CAD build for the part. Positions are in the model's coordinates, mm. Coordinates: 2 decimals unless noted, no trailing zeros.
1) Wall check: line 1 along X through (y, z) = (8, 0.3); line 2 along Y through (x, z) = (11, 2.3); line 3 along X through (y, z) = (83, 2.3). Give the ranges that are in metal, low to high.
2) Pin check, flat tips, straight feed: pin 1 Ø6 at (x, y) = (99.695, 80.645) entering from +Z; pin 2 Ø3.5 at (x, y) = (99.695, 8.255) entering from +Z; pin 3 Ø5 at (x, y) = (8.255, 80.645) entering from +Z. Stop position of each tip, or through.
3) Two-plate mould, pull along Y, no slides. Class faces 1 (the cylindrical face through (1.449, 87.372, 1.61)), 2 (the cylindrical face through (8.7, 78.8, 0.4)), 3 (the cylindrical face through (1.449, 1.528, 1.61)), 4 (the cylindrical face through (101.094, 9.538, 0.431)): +Y half, -Y half, draft (parallel to the pull), parting line (faces both ways), or undercut.
```python
from build123d import *

# Parameters (mm, degrees)
F0_W           = 107.95
F0_H           = 88.9
F1_DEPTH       = 3.175
F3_D           = 3.7973
F3_CSINK_D     = 7.7978
F3_CSINK_ANGLE = 82
F4_R           = 5.08


with BuildPart() as f1:
    # F0 (on Top) → F1 (new body)
    with BuildSketch(Plane.XY):
        with Locations((53.975, 44.45)):
            Rectangle(F0_W, F0_H)
    extrude(amount=F1_DEPTH)

    # F3 (through all)
    with Locations(Plane.XY.offset(3.175)):
        with Locations((8.255, 80.645), (99.695, 80.645), (99.695, 8.255), (8.255, 8.255)):
            CounterSinkHole(F3_D / 2, F3_CSINK_D / 2, counter_sink_angle=F3_CSINK_ANGLE)

    # F4
    f4_edges = [f1.edges().sort_by_distance(p)[0] for p in [
        (0, 0, 1.5875),
        (107.95, 0, 1.5875),
        (107.95, 88.9, 1.5875),
        (0, 88.9, 1.5875),
    ]]
    fillet(f4_edges, radius=F4_R)


solid = f1.part
```
Data:
1. line 1: x = 0 to 6.37, 10.14 to 97.81, 101.58 to 107.95
1. line 2: y = 0 to 6.73, 9.78 to 79.12, 82.17 to 88.9
1. line 3: x = 0 to 6.18, 10.33 to 97.62, 101.77 to 107.95
2. pin 1: stops at z = 2.14
2. pin 2: passes through
2. pin 3: stops at z = 1.57
3. face 1: +Y half
3. face 2: undercut
3. face 3: -Y half
3. face 4: undercut
